Autodesk Inventor part; units mm, degrees
ref_plane "YZ Plane" through (0, 0, 0) normal (1, 0, 0) x (0, 1, 0)
ref_plane "XZ Plane" through (0, 0, 0) normal (0, 1, 0) x (-1, 0, 0)
ref_plane "XY Plane" through (0, 0, 0) normal (0, 0, 1) x (1, 0, 0)
sketch "Szkic1" plane through (0, 0, 0) normal (0, 1, 0) x (-1, 0, 0)
  line L0 (0, 0) -> (35, 0)
  line L1 (35, 0) -> (35, -30)
  line L2 (35, -30) -> (0, -30)
  line L3 (0, -30) -> (0, 0)
  dimension "d0" = 35
  dimension "d1" = 30
extrude "Wyciągnięcie proste1" add sketch "Szkic1" along normal blind 1
sketch "Szkic2" plane through (0, 1, 0) normal (0, 1, 0) x (1, 0, 0)
  line L0 (-35, 30) -> (-35, 0)
  line L1 (-35, 15) -> (-30, 15)
  circle A0 centre (-30, 15) radius 2
  point P0 (0, 0)
  dimension "d4" = 5
  dimension "d5" = 4
extrude "Wyciągnięcie proste2" cut sketch "Szkic2" against normal blind 1
properties part number "Tank resistive sensor"
The model under review builds one solid part; all positions refer to its coordinate system, in mm. Round coordinates to 2 decimals unless told otherwise and drop trailing zeros. Write each loop counter-clockwise with the first axis right and the second up, starting at its lowest first coordinate (ties: lowest second). Pieces come first, ordered by that corner, then holes. Notation, with made-up numbers: M -10.5,21 L 38.5,21 A5 ccw 38.5,25 Z; hole C 34,76.5 d6. An arc over 180 degrees is marked long. Answer as CSV lines item,"result". Start each with the question number.
Q1. Wall thickness on line 1 along X through (y, z) = (0.45, -15); line 2 along Z through (x, y) = (-30, 0.35); line 3 along Z through (x, y) = (-28.5, 0.15): over which ranges is each line inside the solid? List them lowest first.
Q2. Consider section A-A, the plane x = -30. Give the boundary of the cut face in (y, z), then the cut area to 3 significant figures.
Q3. The part is to be moulded in two halves that separate along X. For faces 1 (the face through (-28.092, 0.507, -15.601)), 2 (the face through (0, 0.5, -15.2)), 3 (the face through (-17.3, 0.5, 0)), 4 (the face through (-35, 0.5, -14.8)), say which applies: +X half, -X half, draft (parallel to the pull), parting line (faces both ways), or undercut.
Q4. Consider section B-B, the plane z = -15. Give the boundary of the cut face in (x, y).
Result set:
1,line 1,"x = -35 to -32, -28 to 0"
1,line 2,"z = -30 to -17, -13 to 0"
1,line 3,"z = -30 to -16.32, -13.68 to 0"
2,outline,"M 0,-30 L 1,-30 L 1,-17 L 0,-17 Z; M 0,-13 L 1,-13 L 1,0 L 0,0 Z"
2,area,"26.0 mm²"
3,face 1,"undercut"
3,face 2,"+X half"
3,face 3,"draft"
3,face 4,"-X half"
4,outline,"M -35,0 L -32,0 L -32,1 L -35,1 Z; M -28,0 L 0,0 L 0,1 L -28,1 Z"
